Part print with two shaded views. Sizes in mm from the minimum x, y, z corner. A direction names the side the tool comes from. Round coordinates to 2 decimals unless told otherwise and drop trailing zeros. Write each loop counter-clockwise with the first axis right and the second up, starting at its lowest first coordinate (ties: lowest second). Pieces come first, ordered by that corner, then holes. Notation, with made-up numbers: (-5.75, 64.5) -> (36.25, 64.5) arc R15 ccw to (36.25, 74.5) -> close; hole circle Ø6 at (1, 20). An arc over 180 degrees is marked (long way). Return JSON: item names as keys, results as strings.
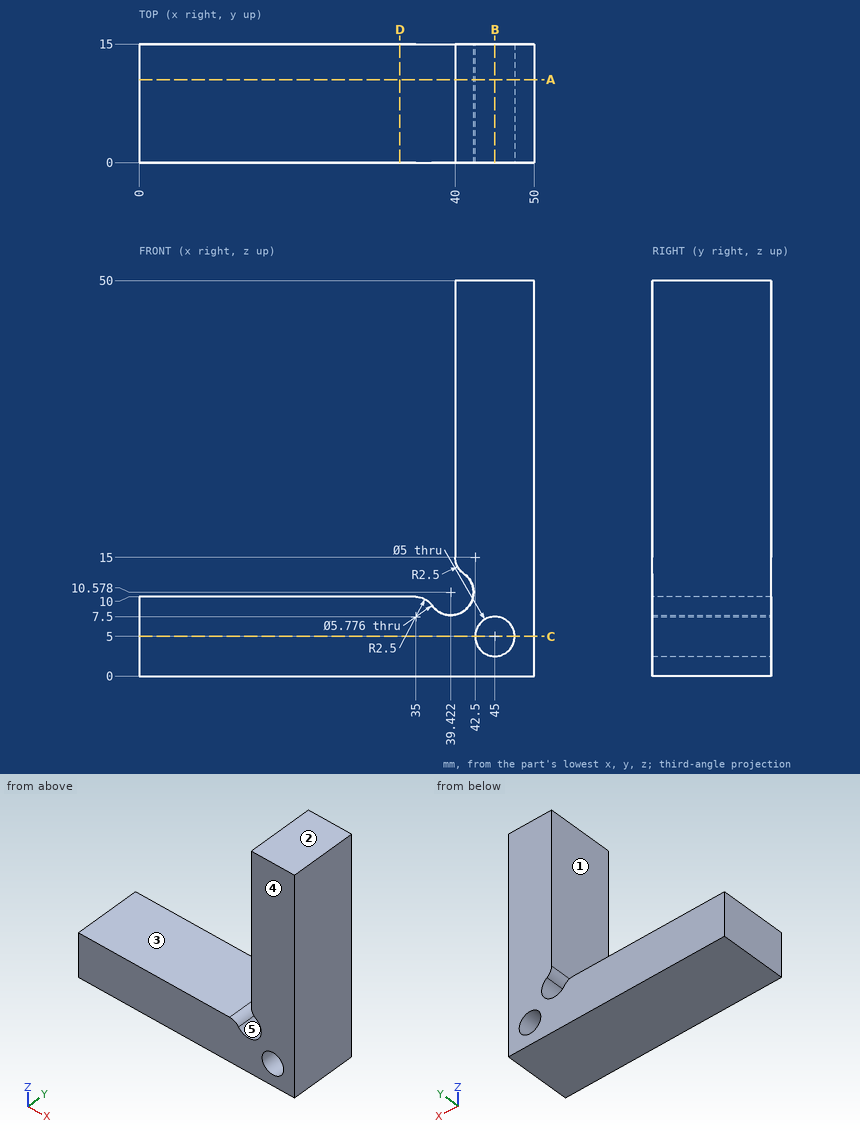
Q1. Saw through at B-B on x = 45. List the corners of the cut face in (y, z), then the cut area to 3 significant figures.
Verdict:
{"outline": "(0, 0) -> (15, 0) -> (15, 2.5) -> (0, 2.5) -> close; (0, 7.5) -> (15, 7.5) -> (15, 50) -> (0, 50) -> close", "area": "675 mm²"}
Q2. Saw through at A-A on y = 10.5. List the corners of the cut face in (x, z) (1 decimal).
Verdict:
{"outline": "(0, 0) -> (50, 0) -> (50, 50) -> (40, 50) -> (40, 15) arc R2.5 ccw to (41.1, 12.9) arc R2.9 cw (long way) to (37.1, 8.9) arc R2.5 ccw to (35, 10) -> (0, 10) -> close; hole circle Ø5 at (45, 5)"}
Q3. Pin check, flat tips, straight feed: pin 1 Ø3 at (x, z) = (17.5, 13) entering from +Y; pin 2 Ø2 at (x, y) = (31, 13) entering from +Z; pin 3 Ø4 at (y, z) = (6, 37) entering from -X. Stop position of each tip, or through.
Verdict:
{"pin 1": "passes through", "pin 2": "stops at z = 10", "pin 3": "stops at x = 40"}
Q4. Wall check: L1, parallel to Z at x = 45, y = 3.5; L2, parallel to Z at x = 10, y = 5.5; L3, parallel to Z at x = 46.5, y = 14. Give the ranges that are in metal, low to high.
Verdict:
{"L1": "z = 0 to 2.5, 7.5 to 50", "L2": "z = 0 to 10", "L3": "z = 0 to 3, 7 to 50"}
Q5. Saw through at D-D on x = 33. List the corners of the cut face in (y, z).
Verdict:
{"outline": "(0, 0) -> (15, 0) -> (15, 10) -> (0, 10) -> close"}
Q6. Two-plate mould, pull along Z, no slides. Class the marked faces 3, 4 and 5: +Z half, -Z half, draft (parallel to the pull), parting line (faces both ways), or undercut.
Verdict:
{"face 3": "+Z half", "face 4": "draft", "face 5": "undercut"}
Q7. Saw through at C-C on z = 5. List the corners of the cut face in (x, y), then the cut area to 3 significant figures.
Verdict:
{"outline": "(0, 0) -> (42.5, 0) -> (42.5, 15) -> (0, 15) -> close; (47.5, 0) -> (50, 0) -> (50, 15) -> (47.5, 15) -> close", "area": "675 mm²"}
Q8. 3-axis set-ups, long thin cutter, end or side, ignore diameter. For the marked faces 1 and 2: which of +Z, -Z, +X, -X, +Y, -Y reach the whole face in a straight line?
Verdict:
{"face 1": "+Z, -X, +Y, -Y", "face 2": "+Z, +X, -X, +Y, -Y"}
